The listing builds one solid part. Answer for the finished solid, in the listing's coordinates (mm). Coordinates: 2 decimals unless noted, no trailing zeros. Order: outer loops, then holes, each group sorted by start corner. A loop starts at its lowest first (then second) coordinate and runs counter-clockwise, first axis right, second up. Notation, with made-up numbers: (16, 35) -> (62, 35) arc R10 cw to (62, 42) -> close; hole circle Ø1 at (50, -15). An arc over 180 degrees is marked (long way). Answer in a Markdown table with one row per item.
```python
from build123d import *

# Parameters (mm, degrees)
SKETCH_1_W          = 6
SKETCH_1_H          = 3
EXTRUDE_1_DEPTH     = 30
SKETCH_2_W          = 1
SKETCH_2_H          = 1.018441017
CUT_EXTRUDE_2_DEPTH = 30
SKETCH_5_W          = 4
SKETCH_5_H          = 1.5
CUT_EXTRUDE_5_DEPTH = 30


with BuildPart() as part:
    # 草圖1 → 填料-伸長1 (new body)
    with BuildSketch(Plane.XY):
        Rectangle(SKETCH_1_W, SKETCH_1_H)
    extrude(amount=EXTRUDE_1_DEPTH)

    # 草圖2 → 除料-伸長2 (cut)
    with BuildSketch(Plane(origin=(0, 0, 0), x_dir=(-1, 0, 0), z_dir=(0, 0, -1))):
        with Locations((0, 0.990779491)):
            Rectangle(SKETCH_2_W, SKETCH_2_H)
    extrude(amount=-CUT_EXTRUDE_2_DEPTH, mode=Mode.SUBTRACT)

    # 草圖5 → 除料-伸長5 (cut)
    with BuildSketch(Plane(origin=(0, 0, 0), x_dir=(-1, 0, 0), z_dir=(0, 0, -1))):
        with Locations((0, -0.25)):
            Rectangle(SKETCH_5_W, SKETCH_5_H)
    extrude(amount=-CUT_EXTRUDE_5_DEPTH, mode=Mode.SUBTRACT)


solid = part.part
```
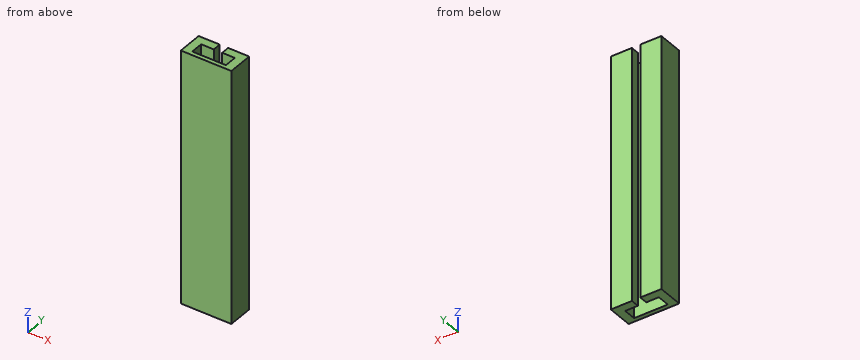
(1) A cutting plane is placed at C-C, the plane z = 26.75. Determine the outline of the cut face in (x, y), then the cut area to 3 significant figures.
Check values:
| item | result |
|---|---|
| outline | (-3, -1.5) -> (3, -1.5) -> (3, 1.5) -> (0.5, 1.5) -> (0.5, 0.5) -> (2, 0.5) -> (2, -1) -> (-2, -1) -> (-2, 0.5) -> (-0.5, 0.5) -> (-0.5, 1.5) -> (-3, 1.5) -> close |
| area | 11.0 mm² |
(2) A cutting plane is placed at B-B, the plane y = -0.35. Determine the outline of the cut face in (x, z).
Check values:
| item | result |
|---|---|
| outline | (-3, 0) -> (-2, 0) -> (-2, 30) -> (-3, 30) -> close; (2, 0) -> (3, 0) -> (3, 30) -> (2, 30) -> close |
(3) A cutting plane is placed at D-D, the plane x = -0.15. Determine the outline of the cut face in (y, z), then the cut area to 3 significant figures.
Check values:
| item | result |
|---|---|
| outline | (-1.5, 0) -> (-1, 0) -> (-1, 30) -> (-1.5, 30) -> close |
| area | 15.0 mm² |
(4) A cutting plane is placed at A-A, the plane x = -1.4. Determine the outline of the cut face in (y, z).
Check values:
| item | result |
|---|---|
| outline | (-1.5, 0) -> (-1, 0) -> (-1, 30) -> (-1.5, 30) -> close; (0.5, 0) -> (1.5, 0) -> (1.5, 30) -> (0.5, 30) -> close |
(5) Find the intervals of material crossed by line 1 along Y through (x, z) = (1.85, 3.5); line 2 along X through (y, z) = (-0.5, 21); line 3 along X through (y, z) = (1.45, 11), in increasing order. Write a range as from..to.
Check values:
| item | result |
|---|---|
| line 1 | -1.5..-1, 0.5..1.5 |
| line 2 | -3..-2, 2..3 |
| line 3 | -3..-0.5, 0.5..3 |
